Autodesk Inventor part; units mm, degrees
ref_plane "YZ Plane" through (0, 0, 0) normal (1, 0, 0) x (0, 1, 0)
ref_plane "XZ Plane" through (0, 0, 0) normal (0, 1, 0) x (-1, 0, 0)
ref_plane "XY Plane" through (0, 0, 0) normal (0, 0, 1) x (1, 0, 0)
sketch "Sketch1" plane through (0, 0, 0) normal (0, 0, 1) x (1, 0, 0)
  circle A0 centre (0, 0) radius 2.4892
  circle A1 centre (-12.7, 8.7884) radius 2.4892
  line L0 (-20.7225, -6.5967) -> (-20.7225, -16.769) construction
  line L1 (-24.8179, -11.6828) -> (-17.0895, -11.6828) construction
  circle A2 centre (-12.7, 21.4884) radius 2.4892
  circle A3 centre (-12.7, 34.1884) radius 2.4892
  circle A4 centre (-12.7, 46.8884) radius 2.4892
  circle A5 centre (12.7, 0) radius 2.4892
  circle A6 centre (25.4, 0) radius 2.4892
  circle A7 centre (38.1, 0) radius 2.4892
  circle A8 centre (0, -12.7) radius 2.4892
  circle A9 centre (12.7, -12.7) radius 2.4892
  circle A10 centre (25.4, -12.7) radius 2.4892
  circle A11 centre (38.1, -12.7) radius 2.4892
  circle A12 centre (-12.7, -3.9116) radius 2.4892
  circle A13 centre (0, -25.4) radius 2.4892
  circle A14 centre (12.7, -25.4) radius 2.4892
  circle A15 centre (25.4, -25.4) radius 2.4892
  circle A16 centre (38.1, -25.4) radius 2.4892
  circle A17 centre (-12.7, -16.6116) radius 2.4892
  circle A18 centre (-12.7, -29.3116) radius 2.4892
  circle A19 centre (-12.7, -42.0116) radius 2.4892
  line L2 (38.1, 0) -> (38.1, 12.7)
  line L3 (38.1, 12.7) -> (44.45, 12.7)
  line L4 (50.8, 12.7) -> (6.35, 12.7)
  line L5 (6.35, -38.1) -> (44.45, -38.1)
  line L6 (50.8, -31.75) -> (50.8, 6.35)
  line L7 (0, -44.45) -> (0, -54.7116)
  line L8 (-25.4, -54.7116) -> (-25.4, 34.1884)
  line L9 (0, 34.1884) -> (0, 19.05)
  line L10 (0, 19.05) -> (6.35, 12.7)
  line L11 (6.35, -38.1) -> (0, -44.45)
  line L12 (44.45, -38.1) -> (50.8, -31.75)
  line L13 (44.45, 12.7) -> (50.8, 6.35)
  circle A20 centre (-12.7, -54.7116) radius 2.4892
  line L14 (-12.7, 21.4884) -> (-12.7, 34.1884)
  line L15 (-12.7, 34.1884) -> (-25.4, 34.1884)
  line L16 (-25.4, 34.1884) -> (-25.4, 34.1884)
  line L17 (-12.7, 34.1884) -> (0, 34.1884)
  line L18 (0, 34.1884) -> (0, 34.1884)
  line L19 (0, -49.5808) -> (0, -67.4116)
  line L20 (0, -67.4116) -> (-25.4, -67.4116)
  line L21 (-25.4, -67.4116) -> (-25.4, -54.7116)
  point P0 (0, -38.1)
  point P1 (0, 12.7)
  point P2 (50.8, -38.1)
  dimension "d0" = 4.9784
  dimension "d1" = 4.9784
  dimension "d2" = 8.7884
  dimension "d3" = 12.7
  dimension "d6" = 12.7
  dimension "d13" = 12.7
  dimension "d28" = 12.7
  dimension "d35" = 12.7
  dimension "d42" = 12.7
  dimension "d43" = 12.7
  dimension "d44" = 50.8
  dimension "d45" = 16.6116
  dimension "d46" = 25.4
  dimension "d47" = 88.9
  dimension "d48" = 6.35
  dimension "d49" = 6.35
  dimension "d50" = 6.35
  dimension "d51" = 6.35
  dimension "d52" = 6.35
  dimension "d53" = 6.35
  dimension "d54" = 6.35
  dimension "d55" = 6.35
  dimension "d60" = 12.7
  dimension "d66" = 12.7
extrude "Extrusion2" add sketch "Sketch1" along normal blind 3.175 contours A3 L17 L9 L10 L4 L3 L13 L6 L12 L5 L11 L7 L19 L20 L21 L8 L15 | A3 L15 L14 | L14 L17 A3
equation "\"d54\" = d52"
equation "\"d55\" = d54"
properties part number "Custom-Underside-L-Gusset" material "Aluminum 6061"
Geometry check sheet. Reference: the model listing, model coordinates, mm. A direction names the side the tool comes from. Coordinates: 2 decimals unless noted, no trailing zeros. Write each loop counter-clockwise with the first axis right and the second up, starting at its lowest first coordinate (ties: lowest second). Pieces come first, ordered by that corner, then holes. Notation, with made-up numbers: M -10.5,-30 L 47.5,-30 A8 cw 47.5,-24 Z; hole C 48.25,-5 d1. An arc over 180 degrees is marked long. Use one line per item in the form item = value. Start each with the question number.
1) Section check B-B on y = -25.4. Enter the section's corners in (x, z) (3 decimals), and give its area (3 significant figures).
2) Thickness scan on probe 1 along Y at (x, z) = (38.1, 2.4); probe 2 along X at (y, z) = (-12, 1.85); probe 3 along X at (y, z) = (-55, 0.35). Record the ranges inside material, lowest first. Write a range as from..to.
3) Release check for a two-part mould opening along X. For faces 3 (the flat face through (0, -56, 2)), 4 (the cylindrical face through (-0.32, -27.87, 1.57)), 5 (the flat face through (4, -16, 0)) record: pulls with the +X half, pulls with the -X half, needs draft (parallel to the pull), parting line crosses it, or undercut.
4) Set-up check for faces 1 (the flat face through (25, -38.1, 2)), 2 (the cylindrical face through (-10.326, -17.359, 1.565)): record each of +Z, -Z, +X, -X, +Y, -Y from which the full face is reachable in a straight line by a thin tool's end or side.
5) Section check C-C on z = 1.2. State how many separate pieces and enclosed holes the cut face has, and give its area (3 significant figures).
6) Go/stop test with flat-tipped pins: pin 1 Ø8 at (x, y) = (25.4, 0) entering from -Z; pin 2 Ø3 at (x, y) = (38.1, 0) entering from -Z; pin 3 Ø1 at (x, z) = (27.5, 1.5) entering from -Y; pin 4 Ø1 at (x, z) = (24, 1) entering from +Y. Record where each tip stops, or that it passes through.
7) Section check A-A on x = 25.4. Enter the section's corners in (y, z) (3 decimals).
Responses:
q1.outline = M -25.4,0 L -2.489,0 L -2.489,3.175 L -25.4,3.175 Z; M 2.489,0 L 10.211,0 L 10.211,3.175 L 2.489,3.175 Z; M 15.189,0 L 22.911,0 L 22.911,3.175 L 15.189,3.175 Z; M 27.889,0 L 35.611,0 L 35.611,3.175 L 27.889,3.175 Z; M 40.589,0 L 50.8,0 L 50.8,3.175 L 40.589,3.175 Z
q1.area = 179 mm2
q2.probe_1 = -38.1..-27.89, -22.91..-15.19, -10.21..-2.49, 2.49..12.7
q2.probe_2 = -25.4..-2.39, 2.39..10.31, 15.09..23.01, 27.79..35.71, 40.49..50.8
q2.probe_3 = -25.4..-15.17, -10.23..0
q3.face_3 = pulls with the +X half
q3.face_4 = undercut
q3.face_5 = needs draft
q4.face_1 = +Z, -Z, +X, -Y
q4.face_2 = +Z, -Z
q5.separate_pieces = 1
q5.enclosed_holes = 19
q5.area = 4,790 mm2
q6.pin_1 = 0
q6.pin_2 = through
q6.pin_3 = -38.1
q6.pin_4 = 12.7
q7.outline = M -38.1,0 L -27.889,0 L -27.889,3.175 L -38.1,3.175 Z; M -22.911,0 L -15.189,0 L -15.189,3.175 L -22.911,3.175 Z; M -10.211,0 L -2.489,0 L -2.489,3.175 L -10.211,3.175 Z; M 2.489,0 L 12.7,0 L 12.7,3.175 L 2.489,3.175 Z
